Geometry check sheet. Reference: the model listing, model coordinates, mm. A direction names the side the tool comes from. Coordinates: 2 decimals unless noted, no trailing zeros. Order: outer loops, then holes, each group sorted by start corner. A loop starts at its lowest first (then second) coordinate and runs counter-clockwise, first axis right, second up. Notation, with made-up numbers: (5, 64.25) -> (64, 64.25) arc R16 ccw to (64, 79.25) -> close; hole circle Ø8 at (10, 65.5). An arc over 180 degrees is marked (long way). Answer in a Markdown table with one row per item. Add a question column.
```python
from build123d import *

# Parameters (mm, degrees)
CROQUIS1_W                                           = 24.75
CROQUIS1_H                                           = 11
SALIENTE_EXTRUIR1_DEPTH                              = 8.25
REFRENTADO_PARA_TORNILLO_CON_CABEZA_HEXA_D           = 3.78
REFRENTADO_PARA_TORNILLO_CON_CABEZA_HEXA_DEPTH       = 8.25
REFRENTADO_PARA_TORNILLO_CON_CABEZA_HEXA_CBORE_D     = 7.2
REFRENTADO_PARA_TORNILLO_CON_CABEZA_HEXA_CBORE_DEPTH = 2.79
DI_METRO_DE_TALADRO_8_5_8_5_1_D                      = 8.5
DI_METRO_DE_TALADRO_8_5_8_5_1_DEPTH                  = 11
CHAFL_N1_SIZE                                        = 1
REDONDEO1_R                                          = 0.5
REDONDEO2_R                                          = 4


with BuildPart() as part:
    # Croquis1 → Saliente-Extruir1 (new body)
    with BuildSketch(Plane(origin=(0, 0, 0), x_dir=(-1, 0, 0), z_dir=(0, 0, -1))):
        Rectangle(CROQUIS1_W, CROQUIS1_H)
    extrude(amount=-SALIENTE_EXTRUIR1_DEPTH)

    # Refrentado para tornillo con cabeza hexagonal de M3.51
    with Locations(Plane.XY.offset(8.25)):
        with Locations((-7.25, 0), (7.25, 0)):
            CounterBoreHole(REFRENTADO_PARA_TORNILLO_CON_CABEZA_HEXA_D / 2, REFRENTADO_PARA_TORNILLO_CON_CABEZA_HEXA_CBORE_D / 2, REFRENTADO_PARA_TORNILLO_CON_CABEZA_HEXA_CBORE_DEPTH, depth=REFRENTADO_PARA_TORNILLO_CON_CABEZA_HEXA_DEPTH)

    # Diámetro de taladro Ø8.5 (8.5)1
    with Locations(Plane(origin=(0, 5.5, 0), x_dir=(1, 0, 0), z_dir=(0, 1, 0))):
        with Locations((0, 0)):
            Hole(DI_METRO_DE_TALADRO_8_5_8_5_1_D / 2, depth=DI_METRO_DE_TALADRO_8_5_8_5_1_DEPTH)

    # Chaflán1
    chafl_n1_edges = [part.edges().sort_by_distance(p)[0] for p in [
        (0, 5.5, 4.25),
        (0, -5.5, 4.25),
    ]]
    chamfer(chafl_n1_edges, length=CHAFL_N1_SIZE)

    # Redondeo1
    redondeo1_edges = [part.edges().sort_by_distance(p)[0] for p in [
        (4.25, 0, 0),
        (-4.25, 0, 0),
    ]]
    fillet(redondeo1_edges, radius=REDONDEO1_R)

    # Redondeo2
    redondeo2_edges = [part.edges().sort_by_distance(p)[0] for p in [
        (-12.375, 5.5, 4.125),
        (-12.375, -5.5, 4.125),
        (12.375, -5.5, 4.125),
        (12.375, 5.5, 4.125),
    ]]
    fillet(redondeo2_edges, radius=REDONDEO2_R)


solid = part.part
```
(1) Cross-section at C-C (x = 0). Enter the section's corners in (y, z).
(2) Scan lines: line 1 along Y through (x, z) = (7.25, 3.75); line 2 along Y through (x, z) = (7.25, 7.6); line 3 along X through (y, z) = (-1, 1.5) (1 decimal). Record each from-to range of solid material in increasing order.
(3) Cross-section at B-B (y = 0). Enter the section's corners in (x, z) (3 decimals), plus the area to 3 significant figures.
(4) Access from +Z, -Z, +X, -X, +Y, -Y to the whole of each face (thin tool, end or side, straight path). Record for faces 1 (the face through (10.684, 1.081, 6.875)), 2 (the face through (11.17, 4.36, 4.18)).
(5) Mould release check, pull along X, two halves, no side actions. Record for faces 3 (the face through (-11.17, 4.36, 4.18)), 4 (the face through (0, -5.5, 6)), 5 (the face through (0.1, 4.66, 4.41)): +X half, -X half, draft (parallel to the pull), parting line (faces both ways), or undercut.
(6) Cross-section at A-A (x = 7.25). Enter the section's corners in (y, z), plus the area to 3 significant figures.
(7) Go/stop test with a flat-tipped pin: P1, Ø6, axis at x = 7, y = 0.5, coming from the +Z side. Record where the tip stops, or that it passes through.
(8) Cross-section at D-D (y = 2.25). Enter the section's corners in (x, z), plus the area to 3 significant figures.
Checks:
| question | item | result |
|---|---|---|
| 1 | outline | (-5.5, 5.25) -> (-4.5, 4.25) -> (4.5, 4.25) -> (5.5, 5.25) -> (5.5, 8.25) -> (-5.5, 8.25) -> close |
| 2 | line 1 | -5.5 to -1.89, 1.89 to 5.5 |
| 2 | line 2 | -5.5 to -3.6, 3.6 to 5.5 |
| 2 | line 3 | -12.4 to -8.9, -5.6 to -4, 4 to 5.6, 8.9 to 12.4 |
| 3 | outline | (-12.375, 0) -> (-9.14, 0) -> (-9.14, 5.46) -> (-10.85, 5.46) -> (-10.85, 8.25) -> (-12.375, 8.25) -> close; (-5.36, 0) -> (-4.724, 0) arc R0.5 ccw to (-4.226, 0.447) arc R4.25 cw to (4.226, 0.447) arc R0.5 ccw to (4.724, 0) -> (5.36, 0) -> (5.36, 5.46) -> (3.65, 5.46) -> (3.65, 8.25) -> (-3.65, 8.25) -> (-3.65, 5.46) -> (-5.36, 5.46) -> close; (9.14, 0) -> (12.375, 0) -> (12.375, 8.25) -> (10.85, 8.25) -> (10.85, 5.46) -> (9.14, 5.46) -> close |
| 3 | area | 94.3 mm² |
| 4 | face 1 | +Z |
| 4 | face 2 | +Z, -Z, +X, +Y |
| 5 | face 3 | -X half |
| 5 | face 4 | draft |
| 5 | face 5 | undercut |
| 6 | outline | (-5.5, 0) -> (-1.89, 0) -> (-1.89, 5.46) -> (-3.6, 5.46) -> (-3.6, 8.25) -> (-5.5, 8.25) -> close; (1.89, 0) -> (5.5, 0) -> (5.5, 8.25) -> (3.6, 8.25) -> (3.6, 5.46) -> (1.89, 5.46) -> close |
| 6 | area | 50.0 mm² |
| 7 | P1 | z = 5.46 |
| 8 | outline | (-12.3, 0) -> (-4.72, 0) arc R0.5 ccw to (-4.23, 0.45) arc R4.25 cw to (4.23, 0.45) arc R0.5 ccw to (4.72, 0) -> (12.3, 0) -> (12.3, 8.25) -> (10.06, 8.25) -> (10.06, 5.46) -> (4.44, 5.46) -> (4.44, 8.25) -> (-4.44, 8.25) -> (-4.44, 5.46) -> (-10.06, 5.46) -> (-10.06, 8.25) -> (-12.3, 8.25) -> close |
| 8 | area | 143 mm² |
